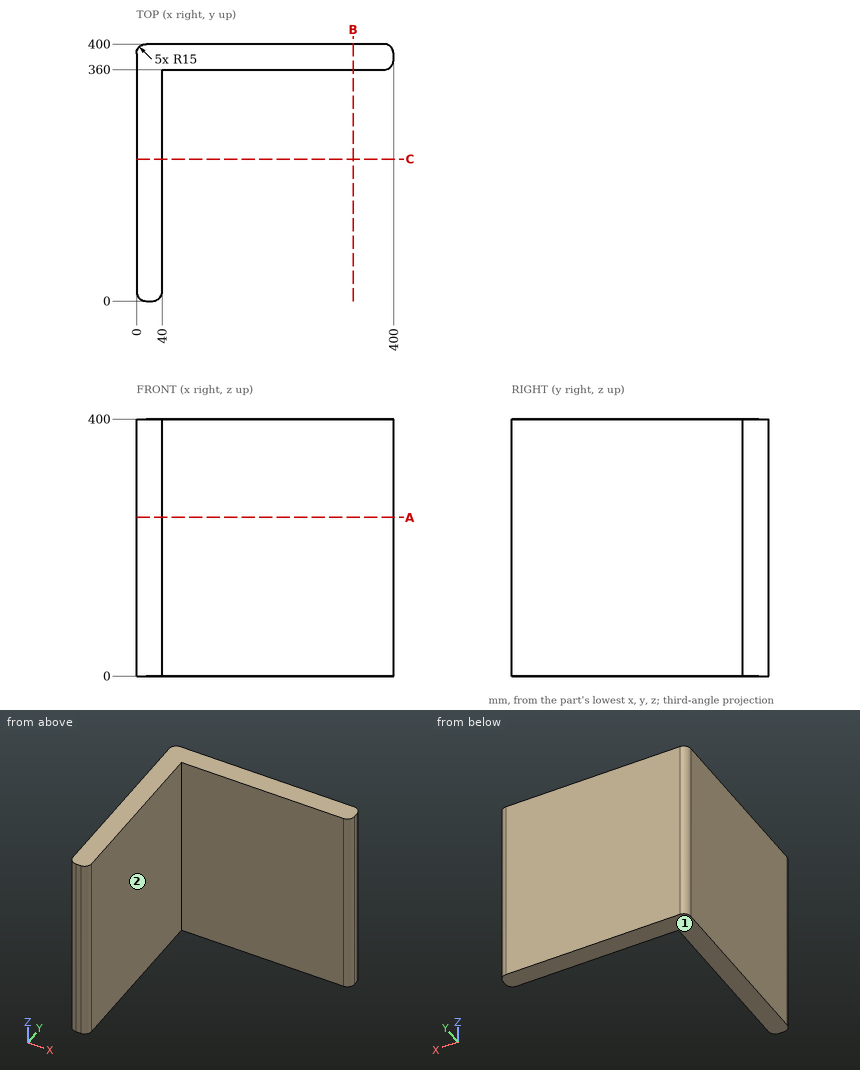
Check sheet for the drawn part. Datum: minimum x, y, z corner. Units: mm. A direction names the side the tool comes from. Round coordinates to 2 decimals unless told otherwise and drop trailing zeros. Write each loop counter-clockwise with the first axis right and the second up, starting at its lowest first coordinate (ties: lowest second). Pieces come first, ordered by that corner, then holes. Notation, with made-up numbers: (51.25, -3) -> (83.25, -3) arc R35 ccw to (83.25, 32) -> close; hole circle Ø3 at (80, 22.25). An arc over 180 degrees is marked (long way). Put each result on its own line as item: value.
(1) Material ranges on line 1 (X direction, y = 121, z = 335); line 2 (Y direction, x = 334, z = 217); line 3 (X direction, y = 367, z = 254.5), recorded low to high.
Values found:
line 1: x = 0 to 40
line 2: y = 360 to 400
line 3: x = 0 to 397.69
(2) Tool access check on the marked faces 1 and 2. Record the directions out of +Z, -Z, +X, -X, +Y, -Y that give a thin tool (end or side, any length) a straight path to the whole face; none if there is none.
Values found:
face 1: -Z, +X, -X, +Y, -Y
face 2: +Z, -Z, +X, -Y
(3) Go/stop test with flat-tipped pins: pin 1 Ø5 at (y, z) = (107.5, 182.5) entering from -X; pin 2 Ø2 at (y, z) = (280, 251) entering from +X; pin 3 Ø1 at (x, z) = (140, 230) entering from -Y. Record where each tip stops, or that it passes through.
Values found:
pin 1: stops at x = 0
pin 2: stops at x = 40
pin 3: stops at y = 360
(4) Sectioned sample at C-C (y = 221). Enter the section's corners in (x, z), plus the area to 3 significant figures.
Values found:
outline: (0, 0) -> (40, 0) -> (40, 400) -> (0, 400) -> close
area: 16,000 mm^2
(5) Sectioned sample at A-A (z = 247). Enter the section's corners in (x, y).
Values found:
outline: (0, 15) arc R15 ccw to (15, 0) -> (25, 0) arc R15 ccw to (40, 15) -> (40, 360) -> (385, 360) arc R15 ccw to (400, 375) -> (400, 385) arc R15 ccw to (385, 400) -> (15, 400) arc R15 ccw to (0, 385) -> close
(6) Sectioned sample at B-B (x = 337). Enter the section's corners in (y, z).
Values found:
outline: (360, 0) -> (400, 0) -> (400, 400) -> (360, 400) -> close
